Read the model definition and answer for the solid it produces. Units are mm, in the model's axes. Face numbers are marked on the shaded views. A direction names the side the tool comes from. Round coordinates to 2 decimals unless told otherwise and drop trailing zeros. Loops run counter-clockwise (first coordinate to the right, second up) from the corner with the lowest first, then second, coordinate; pieces in that order, holes last. Notation, with made-up numbers: (47.25, 60) - (81.25, 60) arc R33 ccw to (81.25, 90) - close; hole circle Ø7 at (-1, -33). An arc over 180 degrees is marked (long way). Use CSV: the item, a comma, the result in double quotes. Start each with the question number.
1. Find section B-B (x = 32.5). Give the vertices of the cut face in (y, z), and give its area (3 significant figures).
2. Find section A-A (y = 27.5). Give the vertices of the cut face in (x, z), and give its area (3 significant figures).
3. Determine the mould class of the marked faces 6, 7 and 8 for opening direction X: +X half, -X half, draft (parallel to the pull), parting line (faces both ways), or undercut.
4. A tool of negligible diameter and unlimited length cuts with its end or side. For the marked faces 1, 2, 3, 4 and 5, from which of +Z, -Z, +X, -X, +Y, -Y can it reach the whole face along a straight path? Write none if from no direction.
5. Consider line 1 along Z through (x, y) = (43, 7.5); line 2 along X through (y, z) = (10, -37); line 3 along Y through (x, z) = (30.5, -3). Determine where each line is inside the solid, lowest interval first.
6. Given pin 1 Ø5.5 at (y, z) = (21.5, -37.5) entering from +X; pin 2 Ø3 at (x, y) = (33, 13.5) entering from +Z; pin 3 Ø11 at (x, z) = (36.5, -6.5) entering from +Y, each flat-ended and moving along its own axis, determine where each tip first touches the part or whether it passes through.
7. Find section C-C (z = -7.5). Give the vertices of the cut face in (x, y).
8. Find section D-D (y = 32). Give the vertices of the cut face in (x, z).
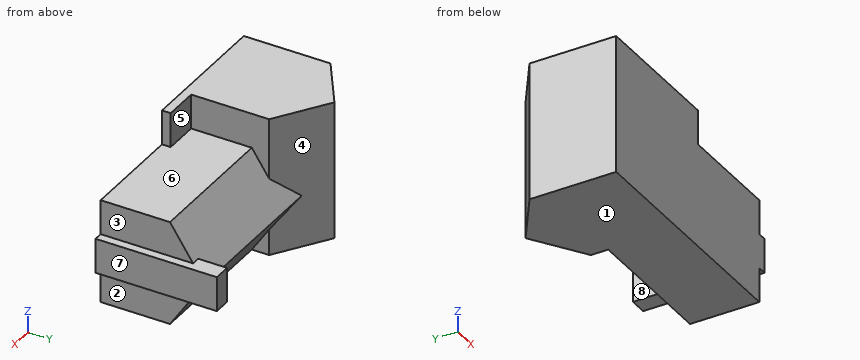
from build123d import *

# Parameters (mm, degrees)
SKETCH1_W                = 30
SKETCH1_H                = 40
BOSS_EXTRUDE1_DEPTH      = 25
BOSS_EXTRUDE2_DEPTH      = 40
SKETCH3_W                = 10
SKETCH3_H                = 40
BOSS_EXTRUDE3_DEPTH      = 2.5
SKETCH4_W                = 30
SKETCH4_H                = 20
BOSS_EXTRUDE4_DEPTH      = 40
BOSS_EXTRUDE5_DEPTH      = 55
SKETCH6_W                = 10
SKETCH6_H                = 35
BOSS_EXTRUDE7_DEPTH      = 2.5
BOSS_EXTRUDE7_DEPTH_BACK = 2.5


with BuildPart() as part:
    # Sketch1 → Boss-Extrude1 (new body)
    with BuildSketch(Plane(origin=(0, 0, 0), x_dir=(1, 0, 0), z_dir=(0, 1, 0))):
        with Locations((15, 20)):
            Rectangle(SKETCH1_W, SKETCH1_H)
    extrude(amount=BOSS_EXTRUDE1_DEPTH)

    # Sketch2 → Boss-Extrude2 (add)
    with BuildSketch(Plane.XY):
        Polygon((15, 25), (30, 25), (15, 35), (0, 25), align=None)
    extrude(amount=-BOSS_EXTRUDE2_DEPTH)

    # Sketch3 → Boss-Extrude3 (add)
    with BuildSketch(Plane(origin=(0, 0, 0), x_dir=(-1, 0, 0), z_dir=(0, -1, 0))):
        with Locations((-35, 20)):
            Rectangle(SKETCH3_W, SKETCH3_H)
    extrude(amount=-BOSS_EXTRUDE3_DEPTH)

    # Sketch4 → Boss-Extrude4 (add)
    with BuildSketch(Plane(origin=(30, 0, 0), x_dir=(0, 0, -1), z_dir=(1, 0, 0))):
        with Locations((25, 10)):
            Rectangle(SKETCH4_W, SKETCH4_H)
    extrude(amount=BOSS_EXTRUDE4_DEPTH)

    # Sketch5 → Boss-Extrude5 (add)
    with BuildSketch(Plane(origin=(70, 0, 0), x_dir=(0, 0, -1), z_dir=(1, 0, 0))):
        Polygon((25, 20), (10, 20), (25, 30), (40, 20), align=None)
    extrude(amount=-BOSS_EXTRUDE5_DEPTH)

    # Sketch6 → Boss-Extrude7 (add, two sides)
    with BuildSketch(Plane(origin=(70, 0, 0), x_dir=(0, 0, -1), z_dir=(1, 0, 0))) as boss_extrude7_sk:
        with Locations((25, 17.5)):
            Rectangle(SKETCH6_W, SKETCH6_H)
    extrude(amount=BOSS_EXTRUDE7_DEPTH)
    extrude(boss_extrude7_sk.sketch, amount=-BOSS_EXTRUDE7_DEPTH_BACK)


solid = part.part
Filled sheet:
1,outline,"(0, -40) - (20, -40) - (30, -25) - (20, -10) - (2.5, -10) - (2.5, 0) - (0, 0) - close"
1,area,"775 mm²"
2,outline,"(3.75, -40) - (26.25, -40) - (26.25, -28.75) - (67.5, -28.75) - (67.5, -30) - (72.5, -30) - (72.5, -20) - (67.5, -20) - (67.5, -21.25) - (26.25, -21.25) - (26.25, 0) - (3.75, 0) - close"
2,area,"1,260 mm²"
3,face 6,"draft"
3,face 7,"+X half"
3,face 8,"undercut"
4,face 1,"-Z, +X, -X, +Y, -Y"
4,face 2,"-Z, +X, +Y, -Y"
4,face 3,"+Z, +X, +Y, -Y"
4,face 4,"+Y"
4,face 5,"+Z, +X, +Y"
5,line 1,"z = -40 to -10"
5,line 2,"x = 0 to 70"
5,line 3,"y = 0 to 2.5"
6,pin 1,"stops at x = 70"
6,pin 2,"stops at z = -10"
6,pin 3,"stops at y = 21.33"
7,outline,"(0, 0) - (40, 0) - (40, 2.5) - (30, 2.5) - (30, 25) - (15, 35) - (0, 25) - close"
8,outline,"(10.5, -40) - (19.5, -40) - (19.5, 0) - (10.5, 0) - close; (67.5, -30) - (72.5, -30) - (72.5, -20) - (67.5, -20) - close"
